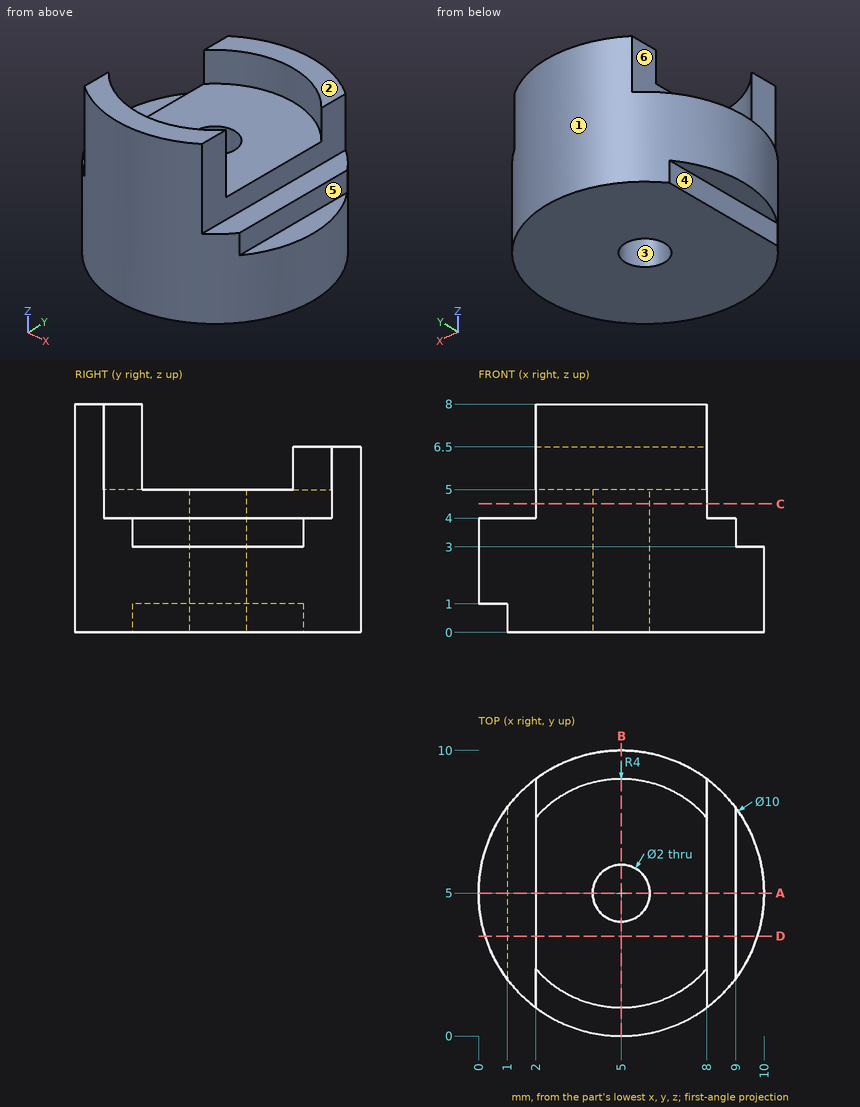
For this review, use the dimensioned drawing (mm, ordinates from the lowest corner) and the shaded views. A direction names the side the tool comes from. Round coordinates to 2 decimals unless told otherwise and drop trailing zeros. Order: outer loops, then holes, each group sorted by start corner. A loop starts at its lowest first (then second) coordinate and runs counter-clockwise, first axis right, second up. Notation, with made-up numbers: M 11,45.5 L 50,45.5 A21 cw 50,64.5 Z; hole C 84,10 d7. An arc over 180 degrees is marked long. Use a Markdown table: item, result.
1) Consider section B-B (x = 5). Write out the cut boundary in (y, z).
Report:
| item | result |
|---|---|
| outline | M 0,0 L 4,0 L 4,5 L 1,5 L 1,8 L 0,8 Z; M 6,0 L 10,0 L 10,6.5 L 9,6.5 L 9,5 L 6,5 Z |
2) Insertion check: pin 1 (2 mm diameter, centred on y = 1.5, z = 4, fed in from -X); pin 2 (0.5 mm diameter, centred on y = 4.5, z = 3.5, fed in from +X); pin 3 (1.5 mm diameter, centred on x = 3, z = 1, fed in from +Y); pin 4 (1.5 mm diameter, centred on x = 2.5, y = 4, fed in from -Z). Each pin has a flat end and moves straight along its axis. Give the tip position at first contact, or say it passes through.
Report:
| item | result |
|---|---|
| pin 1 | x = 0.67 |
| pin 2 | x = 9 |
| pin 3 | y = 9.84 |
| pin 4 | z = 0 |
3) Consider section A-A (y = 5). Write out the cut boundary in (x, z).
Report:
| item | result |
|---|---|
| outline | M 0,1 L 1,1 L 1,0 L 4,0 L 4,5 L 2,5 L 2,4 L 0,4 Z; M 6,0 L 10,0 L 10,3 L 9,3 L 9,4 L 8,4 L 8,5 L 6,5 Z |
4) Wall thickness on line 1 along Y through (x, z) = (5, 3.6); line 2 along Y through (x, z) = (5, 7.25): over which ranges is each line inside the solid? List them lowest first. Write a range as [from, to].
Report:
| item | result |
|---|---|
| line 1 | [0, 4], [6, 10] |
| line 2 | [0, 1] |
5) Tool access review of the marked faces 4, 5 and 6: name each direction out of +Z, -Z, +X, -X, +Y, -Y from which nothing blocks a thin tool from reaching the whole face with its end or side.
Report:
| item | result |
|---|---|
| face 4 | -Z, -X, +Y, -Y |
| face 5 | +Z, +X, +Y, -Y |
| face 6 | +Z, -X, +Y, -Y |
6) Draft analysis for pull direction Y (two halves, no side actions). For the marked faces 1, 2 and 3, state which applies: released by +Y, released by -Y, zero draft, split by the parting line, or undercut.
Report:
| item | result |
|---|---|
| face 1 | split by the parting line |
| face 2 | zero draft |
| face 3 | undercut |
7) Consider section C-C (z = 4.5). Write out the cut boundary in (x, y), then the cut area to 3 significant figures.
Report:
| item | result |
|---|---|
| outline | M 2,1 A5 ccw 8,1 L 8,9 A5 ccw 2,9 Z; hole C 5,5 d2 |
| area | 53.0 mm^2 |
8) Consider section D-D (y = 3.5). Write out the cut boundary in (x, z), then the cut area to 3 significant figures.
Report:
| item | result |
|---|---|
| outline | M 0.23,1 L 1,1 L 1,0 L 9.77,0 L 9.77,3 L 9,3 L 9,4 L 8,4 L 8,5 L 2,5 L 2,4 L 0.23,4 Z |
| area | 42.6 mm^2 |
